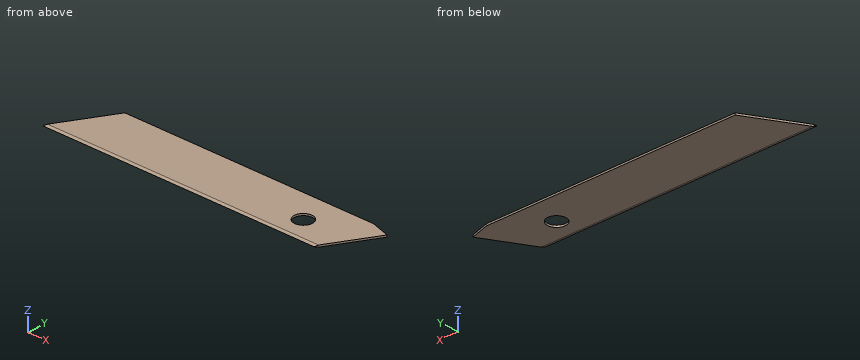
```python
from build123d import *

# Parameters (mm, degrees)
SKETCH_1_R               = 1.5
EXTRUDE_1_DEPTH          = 0.15
CUT_EXTRUDE_1_DEPTH      = 13
CUT_EXTRUDE_1_DEPTH_BACK = 80.3
CUT_EXTRUDE_2_DEPTH      = 1.3


with BuildPart() as part:
    # 草图1 → 凸台-拉伸1 (new body, symmetric)
    with BuildSketch(Plane.XY):
        with BuildLine():
            Line((-74.5, -4), (5.5, -4))
            Line((5.5, -4), (10.132667282, 4.024015107))
            Line((10.132667282, 4.024015107), (7.009129504, 5))
            Line((7.009129504, 5), (-65.987869266, 5))
            ThreePointArc((-65.987869266, 5), (-67.885405091, 4.344282156), (-69.867332718, 4.024015107))
            Line((-69.867332718, 4.024015107), (-74.5, -4))
        make_face()
        Circle(SKETCH_1_R, mode=Mode.SUBTRACT)
    extrude(amount=EXTRUDE_1_DEPTH, both=True)

    # 草图3 → 切除-拉伸1 (cut, two sides)
    with BuildSketch(Plane(origin=(0, 0, 0), x_dir=(0, 0, -1), z_dir=(1, 0, 0))) as cut_extrude_1_sk:
        Polygon((0, -4), (-0.15, -3.5), (-0.747270974, -4.330450708), (0.60266722, -4.330450708), (0.15, -3.5), align=None)
    extrude(amount=CUT_EXTRUDE_1_DEPTH, mode=Mode.SUBTRACT)
    extrude(cut_extrude_1_sk.sketch, amount=-CUT_EXTRUDE_1_DEPTH_BACK, mode=Mode.SUBTRACT)

    # 草图7 → 切除-拉伸2 (cut, through all)
    with BuildSketch(Plane.XY.offset(0.15)):
        Polygon((-30.476363603, 11.629396709), (-39.5, -4), (-74.5, -4), (-62.953845349, 15.998526488), align=None)
    extrude(amount=-CUT_EXTRUDE_2_DEPTH, mode=Mode.SUBTRACT)


solid = part.part
```
The model under review builds one solid part; all positions refer to its coordinate system, in mm. Round coordinates to 2 decimals unless told otherwise and drop trailing zeros. Write each loop counter-clockwise with the first axis right and the second up, starting at its lowest first coordinate (ties: lowest second). Pieces come first, ordered by that corner, then holes. Notation, with made-up numbers: (80.5, 86) - (89.5, 86) arc R5 ccw to (89.5, 90) - close; hole circle Ø6 at (-33, 23). An arc over 180 degrees is marked (long way). Answer as CSV lines item,"result". Start each with the question number.
(1) We need section D-D on y = 2.5. State the section outline as (x, z) points.
(2) We need section A-A on x = 0. State the section outline as (y, z) points, plus the area to 4 significant figures.
(3) We need section C-C on z = -0.1. State the section outline as (x, y) points.
(4) To check wall thickness, follow line 1 (X direction, y = -1, z = -0.05); line 2 (X direction, y = -0.5, z = 0.1); line 3 (X direction, y = -2.75, z = 0). State the ranges of each line that lie inside material, in increasing order.
(5) We need section B-B on y = 0. State the section outline as (x, z) points.
Worked answers:
1,outline,"(-35.75, -0.15) - (9.25, -0.15) - (9.25, 0.15) - (-35.75, 0.15) - close"
2,outline,"(-4, 0) - (-3.5, -0.15) - (-1.5, -0.15) - (-1.5, 0.15) - (-3.5, 0.15) - close; (1.5, -0.15) - (5, -0.15) - (5, 0.15) - (1.5, 0.15) - close"
2,area,"1.725 mm²"
3,outline,"(-39.31, -3.67) - (5.69, -3.67) - (10.13, 4.02) - (7.01, 5) - (-34.3, 5) - close; hole circle Ø3 at (0, 0)"
4,line 1,"-37.77 to -1.12, 1.12 to 7.23"
4,line 2,"-37.48 to -1.41, 1.41 to 7.52"
4,line 3,"-38.78 to 6.22"
5,outline,"(-37.19, -0.15) - (-1.5, -0.15) - (-1.5, 0.15) - (-37.19, 0.15) - close; (1.5, -0.15) - (7.81, -0.15) - (7.81, 0.15) - (1.5, 0.15) - close"
